Autodesk Inventor part; units mm, degrees
ref_plane "Work Plane2" through (0, 63.5, 0) normal (0, -1, 0) x (1, 0, 0)
ref_plane "YZ Plane" through (0, 0, 0) normal (1, 0, 0) x (0, 1, 0)
ref_plane "XZ Plane" through (0, 0, 0) normal (0, 1, 0) x (-1, 0, 0)
sketch "Sketch1" plane through (0, 0, 0) normal (0, 1, 0) x (-1, 0, 0)
  circle A0 centre (0, 0) radius 4
  dimension "d0" = 8
extrude "Extrusion1" add sketch "Sketch1" along normal blind 84.7
ref_plane "Work Plane2" through (0, 63.5, 0) normal (0, -1, 0) x (1, 0, 0)
ref_plane "Work Plane1" through (0, 8, 0) normal (0, -1, 0) x (1, 0, 0)
sketch "Sketch3" plane through (0, 0, 0) normal (0, 0, 1) x (1, 0, 0)
  line L0 (4, 84.7) -> (-4, 84.7)
  line L1 (4, 0) -> (-4, 0)
  line L2 (4, 84.7) -> (-4, 84.7)
  line L3 (4, 0) -> (-4, 0)
  line L4 (4, 63.5) -> (-4, 63.5)
  line L5 (3.6004, 63.5) -> (4.0004, 63.5)
  line L6 (4.0004, 63.5) -> (4.0004, 64.4)
  line L7 (4.0004, 64.4) -> (3.6004, 64.4)
  line L8 (3.6004, 64.4) -> (3.6004, 63.5)
  line L9 (0, -16.94) -> (0, 101.64)
  line L10 (-4, 8) -> (4.0004, 8)
  line L11 (4.0004, 8) -> (3.6004, 8)
  line L12 (3.6004, 8) -> (3.6004, 7.1)
  line L13 (3.6004, 7.1) -> (4.0004, 7.1)
  line L14 (4.0004, 7.1) -> (4.0004, 8)
  point P0 (0, 0)
  dimension "d7" = 63.5
  dimension "d8" = 0.4
  dimension "d9" = 0.9
  dimension "d12" = 8
  dimension "d13" = 0.4
  dimension "d14" = 0.9
revolve "Revolution2" cut sketch "Sketch3" angle 360 about axis through (0, -10, 0) along (0, 1, 0)
properties part number "FlipperRoundShaft"
Geometry check sheet. Reference: the model listing, model coordinates, mm. A direction names the side the tool comes from. Round coordinates to 2 decimals unless told otherwise and drop trailing zeros. Order: outer loops, then holes, each group sorted by start corner. A loop starts at its lowest first (then second) coordinate and runs counter-clockwise, first axis right, second up. Notation, with made-up numbers: (-25, 50.25) - (-9, 50.25) arc R22 cw to (-9, 56.25) - close; hole circle Ø1 at (-39.5, 65). An arc over 180 degrees is marked (long way). One line per question, with ' | ' between items. Start each with the question number.
(1) Sectioned sample at C-C on y = 30. Record the cut outline in (x, z), and give its area (3 significant figures).
(2) Sectioned sample at A-A on x = 2.5. Record the cut outline in (y, z), and give its area (3 significant figures).
(3) Release check for a two-part mould opening along Y. For faces 1 (the cylindrical face through (0.867, 35.362, 3.905)), 2 (the cylindrical face through (3.434, 7.544, 1.081)), 3 (the flat face through (0, 0, 0)), 4 (the flat face through (0, 84.7, 0)) record: released by +Y, released by -Y, zero draft, split by the parting line, or undercut.
(4) Access from +Z, -Z, +X, -X, +Y, -Y to the whole of each face (thin tool, end or side, straight path). Record for faces 5 (the cylindrical face through (0.867, 3.5, 3.905)), 6 (the cylindrical face through (3.434, 63.944, 1.081)).
(5) Sectioned sample at B-B on z = -2. Record the cut outline in (x, y), and give its area (3 significant figures).
(6) Depth check by flat-ended pin: pin 1 Ø1 at (y, z) = (17, 1.5) entering from -X; pin 2 Ø1.5 at (y, z) = (52, -3) entering from -X; pin 3 Ø1.5 at (y, z) = (67, -2.5) entering from +X. Enter the tip coordinate at first touch or a pass-through.
(7) Thickness scan on L1, parallel to Z at x = -0.25, y = 20.5; L2, parallel to X at y = 49, z = 1.75; L3, parallel to X at y = 55, z = 2. Record the ranges inside material, lowest first. Write a range as [from, to].
Conclusion:
1) outline: circle Ø8 at (0, 0) | area: 50.3 mm2
2) outline: (0, -3.12) - (7.1, -3.12) - (7.1, -2.59) - (8, -2.59) - (8, -3.12) - (63.5, -3.12) - (63.5, -2.59) - (64.4, -2.59) - (64.4, -3.12) - (84.7, -3.12) - (84.7, 3.12) - (64.4, 3.12) - (64.4, 2.59) - (63.5, 2.59) - (63.5, 3.12) - (8, 3.12) - (8, 2.59) - (7.1, 2.59) - (7.1, 3.12) - (0, 3.12) - close | area: 527 mm2
3) face 1: zero draft | face 2: undercut | face 3: released by -Y | face 4: released by +Y
4) face 5: +Y, -Y | face 6: none
5) outline: (-3.46, 0) - (3.46, 0) - (3.46, 7.1) - (2.99, 7.1) - (2.99, 8) - (3.46, 8) - (3.46, 63.5) - (2.99, 63.5) - (2.99, 64.4) - (3.46, 64.4) - (3.46, 84.7) - (-3.46, 84.7) - (-3.46, 64.4) - (-2.99, 64.4) - (-2.99, 63.5) - (-3.46, 63.5) - (-3.46, 8) - (-2.99, 8) - (-2.99, 7.1) - (-3.46, 7.1) - close | area: 585 mm2
6) pin 1: stops at x = -3.87 | pin 2: stops at x = -3.31 | pin 3: stops at x = 3.6
7) L1: z = [-3.99, 3.99] | L2: x = [-3.6, 3.6] | L3: x = [-3.46, 3.46]
